Work out the finished part from the listing and answer in its coordinate system (mm). A direction names the side the tool comes from. Give positions to 0.01 mm unless a question says otherwise; leave off trailing zeros. Order: outer loops, then holes, each group sorted by start corner. A loop starts at its lowest first (then second) coordinate and runs counter-clockwise, first axis right, second up.
```python
from build123d import *
from OCP.BRepAlgoAPI import BRepAlgoAPI_Cut
from OCP.TopTools import TopTools_ListOfShape

# Parameters (mm, degrees)
BOSS_EXTRUDE1_DEPTH = 70
CUT_EXTRUDE4_DEPTH  = 70


with BuildPart() as part:
    # Sketch1 → Boss-Extrude1 (new body)
    with BuildSketch(Plane(origin=(0, 0, 0), x_dir=(0, 0, -1), z_dir=(1, 0, 0))):
        with BuildLine():
            Line((1, 0), (25.334184189, 0))
            ThreePointArc((25.334184189, 0), (26.748397751, 0.585786438), (27.334184189, 2))
            Line((27.334184189, 2), (27.334184189, 77.577100538))
            Line((27.334184189, 77.577100538), (16.217438852, 153.114908847))
            ThreePointArc((16.217438852, 153.114908847), (15.853623852, 153.749510415), (15.155100701, 153.966641506))
            Line((15.155100701, 153.966641506), (14.155100701, 153.893451695))
            ThreePointArc((14.155100701, 153.893451695), (13.447894018, 153.521647944), (13.238751678, 152.750519677))
            Line((13.238751678, 152.750519677), (24.334184189, 77.357531107))
            Line((24.334184189, 77.357531107), (24.334184189, 5))
            ThreePointArc((24.334184189, 5), (23.748397751, 3.585786438), (22.334184189, 3))
            Line((22.334184189, 3), (1, 3))
            ThreePointArc((1, 3), (0.292893219, 2.707106781), (0, 2))
            Line((0, 2), (0, 1))
            ThreePointArc((0, 1), (0.292893219, 0.292893219), (1, 0))
        make_face()
    extrude(amount=BOSS_EXTRUDE1_DEPTH)


with BuildPart() as cut_extrude4_tool:
    # Sketch2 → Cut-Extrude4 (new body)
    with BuildSketch(Plane.XY):
        with BuildLine():
            Line((0, 1), (0, 154.250011553))
            Line((0, 154.250011553), (4, 154.250011553))
            Line((4, 154.250011553), (4, 77.357531107))
            add(Edge.make_bspline(
                [(4, 77.357531107), (4.361118304, 39.105803732), (0, 1)],
                knots=[0, 0, 0, 1, 1, 1], degree=2))
        make_face()
        with BuildLine():
            Line((70, 154.250011553), (66, 154.250011553))
            Line((66, 154.250011553), (66, 77.357531107))
            add(Edge.make_bspline(
                [(66, 77.357531107), (65.638881696, 39.105803732), (70, 1)],
                knots=[0, 0, 0, 1, 1, 1], degree=2))
            Line((70, 1), (70, 154.250011553))
        make_face()
    extrude(amount=-CUT_EXTRUDE4_DEPTH)


with BuildPart() as part_1:
    add(part.part)

    # Cut-Extrude4: cut by cut_extrude4_tool, with a tolerance
    cut_extrude4_stock = TopTools_ListOfShape()
    cut_extrude4_stock.Append(part_1.part.wrapped)
    cut_extrude4_tools = TopTools_ListOfShape()
    cut_extrude4_tools.Append(cut_extrude4_tool.part.wrapped)
    cut_extrude4_cut = BRepAlgoAPI_Cut()
    cut_extrude4_cut.SetArguments(cut_extrude4_stock)
    cut_extrude4_cut.SetTools(cut_extrude4_tools)
    cut_extrude4_cut.SetFuzzyValue(0.00001)
    cut_extrude4_cut.Build()
    add(Compound.cast(cut_extrude4_cut.Shape()).solids(), mode=Mode.REPLACE)


solid = part_1.part
```
1. Straight lines are drawn through the part: probe 1 along Z at (x, y) = (55, 63); probe 2 along X at (y, z) = (83, -25.25); probe 3 along Z at (x, y) = (6, 115.5). For each, find the intervals that lie inside material, in ascending order.
Findings below:
probe 1: z = -27.33 to -24.33
probe 2: x = 4 to 66
probe 3: z = -21.75 to -18.72
2. The mould has two halves that part along Y. Classify faces 1 (the face through (35, 3, -12)), 2 (the face through (35, 42, -24.334)), 3 (the face through (34.566, 114.817, -21.854)), 4 (the face through (4, 116, -20)): pulls with the +Y half, pulls with the -Y half, needs draft (parallel to the pull), parting line crosses it, or undercut.
Findings below:
face 1: undercut
face 2: undercut
face 3: pulls with the +Y half
face 4: needs draft
3. The part is cut by section B-B (y = 87.5). Write down the section's boundary in (x, z), then the cut area to 3 significant figures.
Findings below:
outline: (4, -25.87) - (66, -25.87) - (66, -22.84) - (4, -22.84) - close
area: 188 mm2
4. Given P1, Ø3, axis at x = 34, z = -10, coming from the +Y side; P2, Ø1.5, axis at x = 32.5, y = 132, coming from the +Z side; P3, Ø2, axis at x = 54, y = 92, coming from the +Z side; P4, Ø4, axis at y = 98, z = -17.5, coming from the +X side, each flat-ended and moving along its own axis, determine where each tip first touches the part or whether it passes through.
Findings below:
P1: stops at y = 3
P2: stops at z = -16.18
P3: stops at z = -22.03
P4: passes through
5. Which of the six approach directions +Z, -Z, +X, -X, +Y, -Y give full straight-line access (tool end or side, diameter ignored) to faces 5 (the face through (66, 116, -20)), 6 (the face through (35, 39, -27.334)), 7 (the face through (34.57, 115.58, -18.71))?
Findings below:
face 5: +Z, -Z, +X, +Y
face 6: -Z, +X, -X, +Y, -Y
face 7: +Z, +X, -X
6. The part is cut by section A-A (x = 10.5). Write down the section's boundary in (y, z).
Findings below:
outline: (0, -25.33) arc R2 ccw to (2, -27.33) - (77.58, -27.33) - (153.11, -16.22) arc R1 ccw to (153.97, -15.16) - (153.89, -14.16) arc R1 ccw to (152.75, -13.24) - (77.36, -24.33) - (5, -24.33) arc R2 cw to (3, -22.33) - (3, -1) arc R1 ccw to (2, 0) - (1, 0) arc R1 ccw to (0, -1) - close
